from build123d import *

# Parameters (mm, degrees)
CROQUIS2_W                                           = 76.512018684
CROQUIS2_H                                           = 18.314660831
SALIENTE_EXTRUIR1_DEPTH                              = 10
CROQUIS1_R                                           = 6.5
CROQUIS1_R_2                                         = 2.65
SALIENTE_EXTRUIR2_DEPTH                              = 5
CORTAR_EXTRUIR1_DEPTH                                = 31
CORTAR_EXTRUIR1_DEPTH_BACK                           = 50
CROQUIS4_R                                           = 2.5
REFRENTADO_PARA_TORNILLO_CON_CABEZA_TRON_D           = 5.3
REFRENTADO_PARA_TORNILLO_CON_CABEZA_TRON_CBORE_D     = 11
REFRENTADO_PARA_TORNILLO_CON_CABEZA_TRON_CBORE_DEPTH = 3.7
REFRENTADO_PARA_TORNILLO_CON_CABEZA_2_D              = 5.3
REFRENTADO_PARA_TORNILLO_CON_CABEZA_2_CBORE_D        = 11
REFRENTADO_PARA_TORNILLO_CON_CABEZA_2_CBORE_DEPTH    = 3.7
REFRENTADO_PARA_TORNILLO_CON_CABEZA_3_D              = 5.3
REFRENTADO_PARA_TORNILLO_CON_CABEZA_3_CBORE_D        = 11
REFRENTADO_PARA_TORNILLO_CON_CABEZA_3_CBORE_DEPTH    = 3.7


with BuildPart() as part:
    # Croquis2 → Saliente-Extruir1 (new body)
    with BuildSketch(Plane(origin=(0, 0, 0), x_dir=(1, 0, 0), z_dir=(0, 1, 0))):
        with Locations((0.23849107, 24.625561378)):
            Rectangle(CROQUIS2_W, CROQUIS2_H)
    extrude(amount=SALIENTE_EXTRUIR1_DEPTH)

    # Croquis1 → Saliente-Extruir2 (add)
    # profile 1 of 2: a face of its own
    with BuildSketch(Plane(origin=(0, 0, 0), x_dir=(1, 0, 0), z_dir=(0, 1, 0))):
        with Locations(Location((-30.5, 25.086633895, 0), (0, 0, 270))):
            Circle(CROQUIS1_R)
        with Locations(Location((-30.5, 25.086633895, 0), (0, 0, 270))):
            Circle(CROQUIS1_R_2, mode=Mode.SUBTRACT)
    # profile 2 of 2: a face of its own
    with BuildSketch(Plane(origin=(0, 0, 0), x_dir=(1, 0, 0), z_dir=(0, 1, 0))):
        with Locations(Location((30.5, 25.086633895, 0), (0, 0, 90))):
            Circle(CROQUIS1_R)
        with Locations(Location((30.5, 25.086633895, 0), (0, 0, 270))):
            Circle(CROQUIS1_R_2, mode=Mode.SUBTRACT)
    extrude(amount=-SALIENTE_EXTRUIR2_DEPTH)

    # Croquis4 → Cortar-Extruir1 (cut, two sides: drawn at the far end of the back side and taken through both)
    with BuildSketch(Plane.XZ.offset(-CORTAR_EXTRUIR1_DEPTH_BACK)):
        with Locations(Location((-30.5, -25.086633895, 0), (0, 0, 90))):
            Circle(CROQUIS4_R)
        with Locations(Location((30.5, -25.086633895, 0), (0, 0, 90))):
            Circle(CROQUIS4_R)
    extrude(amount=CORTAR_EXTRUIR1_DEPTH + CORTAR_EXTRUIR1_DEPTH_BACK, mode=Mode.SUBTRACT)

    # Refrentado para tornillo con cabeza tron (through all)
    with Locations(Plane(origin=(-30.5, 10, -25.086633895), x_dir=(0, 0, 1), z_dir=(0, 1, 0))):
        with Locations((0, 0)):
            CounterBoreHole(REFRENTADO_PARA_TORNILLO_CON_CABEZA_TRON_D / 2, REFRENTADO_PARA_TORNILLO_CON_CABEZA_TRON_CBORE_D / 2, REFRENTADO_PARA_TORNILLO_CON_CABEZA_TRON_CBORE_DEPTH)

    # Refrentado para tornillo con cabeza  2 (through all)
    with Locations(Plane(origin=(-30.5, 6.3, -25.086633895), x_dir=(0, 0, 1), z_dir=(0, 1, 0))):
        with Locations((0, 0)):
            CounterBoreHole(REFRENTADO_PARA_TORNILLO_CON_CABEZA_2_D / 2, REFRENTADO_PARA_TORNILLO_CON_CABEZA_2_CBORE_D / 2, REFRENTADO_PARA_TORNILLO_CON_CABEZA_2_CBORE_DEPTH)

    # Refrentado para tornillo con cabeza  3 (through all)
    with Locations(Plane(origin=(30.5, 10, -25.086633895), x_dir=(0, 0, 1), z_dir=(0, 1, 0))):
        with Locations((0, 0)):
            CounterBoreHole(REFRENTADO_PARA_TORNILLO_CON_CABEZA_3_D / 2, REFRENTADO_PARA_TORNILLO_CON_CABEZA_3_CBORE_D / 2, REFRENTADO_PARA_TORNILLO_CON_CABEZA_3_CBORE_DEPTH)


solid = part.part
The model under review builds one solid part; all positions refer to its coordinate system, in mm. A direction names the side the tool comes from. Round coordinates to 2 decimals unless told otherwise and drop trailing zeros. Write each loop counter-clockwise with the first axis right and the second up, starting at its lowest first coordinate (ties: lowest second). Pieces come first, ordered by that corner, then holes. Notation, with made-up numbers: (81.25, 57.25) -> (100.25, 57.25) arc R28 cw to (100.25, 84.25) -> close; hole circle Ø8 at (24.5, 78.25). An arc over 180 degrees is marked (long way). Answer as a JSON object with one key per item and string values.
1. Clearance check with flat-ended pins moving along their axes: pin 1 (5 mm diameter, centred on x = -0.5, z = -24, fed in from -Y); pin 2 (2 mm diameter, centred on x = -28, y = -3, fed in from +Z); pin 3 (5.5 mm diameter, centred on x = -30, z = -27.5, fed in from +Y). State where each tip first meets the part, or that it passes through.
Results found:
{"pin 1": "stops at y = 0", "pin 2": "stops at z = -18.76", "pin 3": "stops at y = 2.6"}
2. The part is to be moulded in two halves that separate along Z. For faces 1 (the face through (0, 5, -33.783)), 2 (the face through (29, 6.3, -28)), 3 (the face through (0, 0, -25)), say which applies: pulls with the +Z half, pulls with the -Z half, needs draft (parallel to the pull), parting line crosses it, or undercut.
Results found:
{"face 1": "pulls with the -Z half", "face 2": "undercut", "face 3": "needs draft"}
3. Machinability: for faces 4 (the face through (-32, 2.6, -28)), 5 (the face through (24.055, -2.465, -24.24)), 6 (the face through (33.3, -5, -25)), which of the approach directions +Z, -Z, +X, -X, +Y, -Y give a long, thin tool a straight path to every point of the face, cutting with its end or side? Answer none if there is none.
Results found:
{"face 4": "+Y", "face 5": "-Y", "face 6": "+Z, -Z, +X, -X, -Y"}
4. We need section B-B on z = -24.5. State the section outline as (x, y) points, and give its area (4 significant figures).
Results found:
{"outline": "(-38.02, 0) -> (-36.97, 0) -> (-36.97, -5) -> (-33.08, -5) -> (-33.08, 2.6) -> (-35.97, 2.6) -> (-35.97, 10) -> (-38.02, 10) -> close; (-27.92, -5) -> (-24.03, -5) -> (-24.03, 0) -> (24.03, 0) -> (24.03, -5) -> (27.92, -5) -> (27.92, 6.3) -> (25.03, 6.3) -> (25.03, 10) -> (-25.03, 10) -> (-25.03, 2.6) -> (-27.92, 2.6) -> close; (33.08, -5) -> (36.97, -5) -> (36.97, 0) -> (38.49, 0) -> (38.49, 10) -> (35.97, 10) -> (35.97, 6.3) -> (33.08, 6.3) -> close", "area": "675.5 mm^2"}
5. We need section A-A on y = -2.75. State the section outline as (x, z) points.
Results found:
{"outline": "circle Ø13 at (-30.5, -25.09); circle Ø13 at (30.5, -25.09); hole circle Ø5.3 at (-30.5, -25.09); hole circle Ø5.3 at (30.5, -25.09)"}
6. To check wall thickness, follow line 1 along X through (y, z) = (-3, -25); line 2 along X through (y, z) = (8.5, -26.75); line 3 along X through (y, z) = (0.75, -27.25). State the ranges of each line that lie inside material, in increasing order.
Results found:
{"line 1": "x = -37 to -33.15, -27.85 to -24, 24 to 27.85, 33.15 to 37", "line 2": "x = -38.02 to -35.74, -25.26 to 25.26, 35.74 to 38.49", "line 3": "x = -38.02 to -32.03, -28.97 to 28.97, 32.03 to 38.49"}
7. We need section C-C on x = 2.5. State the section outline as (y, z) points, and give its area (3 significant figures).
Results found:
{"outline": "(0, -33.78) -> (10, -33.78) -> (10, -15.47) -> (0, -15.47) -> close", "area": "183 mm^2"}
